Source: CAD feature listing. Evaluate the final solid. Frame: model axes, mm. Face numbers are marked on the shaded views. A direction names the side the tool comes from. Coordinates: 2 decimals unless noted, no trailing zeros. Order: outer loops, then holes, each group sorted by start corner. A loop starts at its lowest first (then second) coordinate and runs counter-clockwise, first axis right, second up.
Item 1: Reachability of the marked faces 1 and 2 from +Z, -Z, +X, -X, +Y, -Y: full face, straight path, thin tool, end or side. Return the list, or none.
Item 2: Section B-B on z = -25. Return the cut outline in (x, y) (3 decimals).
Item 3: Ray query, line 1 (X direction, y = 6.5, z = -25); line 2 (Y direction, x = 50, z = -3.4) (3 decimals); line 3 (Y direction, x = 100.5, z = -23). Return the intervals inside material, ascending.
Item 4: Section A-A on x = 10. Return the cut outline in (y, z).
Item 5: Section D-D on z = -14.5. Return the cut outline in (x, y) (3 decimals).
Item 6: Mould query, pull axis X, two halves, no side actions, for the marked faces 3, 4 and 5. Classes: released by +X, released by -X, zero draft, split by the parting line, or undercut.
Item 7: Contact query for flat-ended pins moving along their axis: P1, Ø5.5, axis at x = 48, y = 33, coming from the +Z side; P2, Ø2, axis at x = 40.5, y = 24, coming from the -Z side; P3, Ø2, axis at y = 41.5, z = -10, coming from the -X side. Output: stop coordinate, or through.
Item 8: Section C-C on y = 18.5. Return the cut outline in (x, z), then the cut area to 3 significant figures.
from build123d import *

# Parameters (mm, degrees)
CROQUIS1_W                                           = 150
CROQUIS1_H                                           = 40
SALIENTE_EXTRUIR1_DEPTH                              = 10
SALIENTE_EXTRUIR2_DEPTH                              = 10
CROQUIS3_W                                           = 40
CROQUIS3_H                                           = 3
CORTAR_EXTRUIR1_DEPTH                                = 165.69669092
REFRENTADO_PARA_PERNO_CON_CABEZA_HEXAGON_D           = 9
REFRENTADO_PARA_PERNO_CON_CABEZA_HEXAGON_CBORE_D     = 18.01
REFRENTADO_PARA_PERNO_CON_CABEZA_HEXAGON_CBORE_DEPTH = 5.68
REDONDEO1_R                                          = 8
REDONDEO2_R                                          = 8
REDONDEO3_R                                          = 3
TALADRO_DE_MARGEN_PARA_M71_D                         = 7.6


with BuildPart() as part:
    # Croquis1 → Saliente-Extruir1 (new body)
    with BuildSketch(Plane(origin=(0, 0, 0), x_dir=(1, 0, 0), z_dir=(0, 1, 0))):
        with Locations((75, 20)):
            Rectangle(CROQUIS1_W, CROQUIS1_H)
    extrude(amount=SALIENTE_EXTRUIR1_DEPTH)

    # Croquis2 → Saliente-Extruir2 (add)
    with BuildSketch(Plane.XY):
        with BuildLine():
            Line((30, 0), (30, 35))
            ThreePointArc((30, 35), (50, 55), (70, 35))
            Line((70, 35), (70, 0))
            Line((70, 0), (30, 0))
        make_face()
    extrude(amount=-SALIENTE_EXTRUIR2_DEPTH)

    # Croquis3 → Cortar-Extruir1 (cut, through all)
    with BuildSketch(Plane.XY):
        with Locations((50, 1.5)):
            Rectangle(CROQUIS3_W, CROQUIS3_H)
    extrude(amount=-CORTAR_EXTRUIR1_DEPTH, mode=Mode.SUBTRACT)

    # Refrentado para perno con cabeza hexagonal de M81 (through all)
    with Locations(Plane.XY):
        with Locations((50, 35)):
            CounterBoreHole(REFRENTADO_PARA_PERNO_CON_CABEZA_HEXAGON_D / 2, REFRENTADO_PARA_PERNO_CON_CABEZA_HEXAGON_CBORE_D / 2, REFRENTADO_PARA_PERNO_CON_CABEZA_HEXAGON_CBORE_DEPTH)

    # Redondeo1
    # the kernel refuses this fillet: 8 mm, written as the material it adds along each edge
    with BuildSketch(Plane(origin=(70, 3, 0), x_dir=(-1, 0, 0), z_dir=(0, 0, -1))) as redondeo1_piece_1:
        with BuildLine():
            CenterArc((6.244997998, -8), REDONDEO1_R, 90, 51.317812547)
            Line((0, -3), (-0.12489996, -2.9))
            ThreePointArc((-0.12489996, -2.9), (-0.16, -1.5), (-0.16, 0))
            Line((-0.16, 0), (0, 0.16))
            Line((0, 0.16), (6.244997998, 0.16))
            Line((6.244997998, 0.16), (6.244997998, 0))
        make_face()
    extrude(amount=40)
    with BuildSketch(Plane(origin=(30, 3, 0), x_dir=(0, -1, 0), z_dir=(0, 0, -1))) as redondeo1_piece_2:
        with BuildLine():
            CenterArc((8, -6.244997998), REDONDEO1_R, 128.682187453, 51.317812547)
            Line((0, -6.244997998), (-0.16, -6.244997998))
            Line((-0.16, -6.244997998), (-0.16, 0))
            Line((-0.16, 0), (0, 0.16))
            ThreePointArc((0, 0.16), (1.5, 0.16), (2.9, 0.12489996))
            Line((2.9, 0.12489996), (3, 0))
        make_face()
    extrude(amount=40)

    # Redondeo2
    redondeo2_edges = [part.edges().sort_by_distance(p)[0] for p in [
        (0, 5, -40),
        (0, 5, 0),
        (150, 5, 0),
        (150, 5, -40),
    ]]
    fillet(redondeo2_edges, radius=REDONDEO2_R)

    # Redondeo3
    redondeo3_edges = [part.edges().sort_by_distance(p)[0] for p in [
        (106, 10, 0),
        (30, 22.5, -10),
        (30, 10, -5),
        (50, 55, -10),
        (70, 10, -5),
        (70, 22.5, -10),
        (50, 10, -10),
        (70, 22.5, 0),
        (50, 55, 0),
        (30, 22.5, 0),
        (150, 10, -20),
        (19, 10, 0),
        (75, 10, -40),
        (0, 10, -20),
        (2.343145751, 10, -2.343145751),
        (2.343145751, 10, -37.656854249),
        (147.656854249, 10, -37.656854249),
        (147.656854249, 10, -2.343145751),
    ]]
    fillet(redondeo3_edges, radius=REDONDEO3_R)

    # Taladro de margen para M71 (through all)
    with Locations(Plane(origin=(0, 10, 0), x_dir=(1, 0, 0), z_dir=(0, 1, 0))):
        with Locations((140, 25), (10, 25)):
            Hole(TALADRO_DE_MARGEN_PARA_M71_D / 2)


solid = part.part
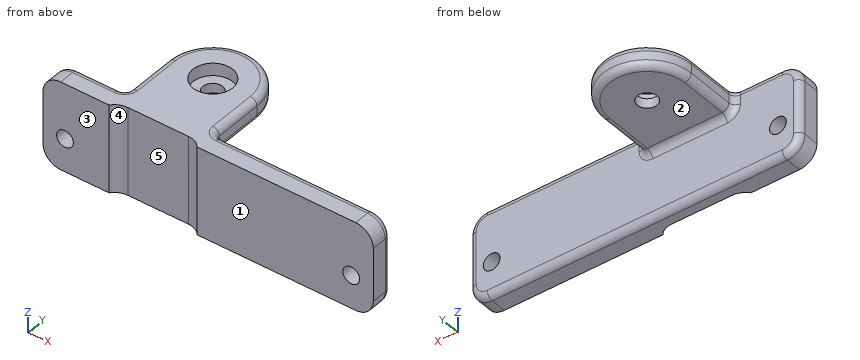
Answer list:
1. face 1: +Z, -Z, +X, -X, -Y
1. face 2: -Z, +X, -X, +Y
2. outline: (0, 0) - (6.2, 0) - (6.2, 10) - (3, 10) arc R3 ccw to (0, 7) - close; (13.8, 0) - (30, 0) arc R8 cw to (36.245, 3) - (63.755, 3) arc R8 cw to (70, 0) - (136.2, 0) - (136.2, 10) - (13.8, 10) - close; (143.8, 0) - (150, 0) - (150, 7) arc R3 ccw to (147, 10) - (143.8, 10) - close
3. line 1: x = 0 to 6.2, 13.8 to 136.2, 143.8 to 150
3. line 2: y = 3 to 25.995, 44.005 to 55
3. line 3: y = 0 to 10
4. outline: (0, -40) - (7, -40) arc R3 ccw to (10, -37) - (10, -28.8) - (0, -28.8) - close; (0, -21.2) - (10, -21.2) - (10, -3) arc R3 ccw to (7, 0) - (0, 0) - close
5. outline: (0, 0) - (30, 0) arc R8 cw to (36.245, 3) - (63.755, 3) arc R8 cw to (70, 0) - (150, 0) - (150, 7) arc R3 ccw to (147, 10) - (3, 10) arc R3 ccw to (0, 7) - close
6. face 3: zero draft
6. face 4: undercut
6. face 5: undercut
7. P1: stops at z = -5.68
7. P2: stops at z = -10
7. P3: stops at x = 31.83
8. outline: (30, -7) arc R3 ccw to (33, -10) - (67, -10) arc R3 ccw to (70, -7) - (70, -3) arc R3 ccw to (67, 0) - (33, 0) arc R3 ccw to (30, -3) - close
8. area: 392 mm2
